from build123d import *

# Parameters (mm, degrees)
SKETCH1_W           = 4
SKETCH1_H           = 4
BOSS_EXTRUDE1_DEPTH = 12
CHAMFER3_SIZE       = 1
CHAMFER4_SIZE       = 1


with BuildPart() as part:
    # Sketch1 → Boss-Extrude1 (new body)
    with BuildSketch(Plane(origin=(0, 0, 0), x_dir=(1, 0, 0), z_dir=(0, 1, 0))):
        Rectangle(SKETCH1_W, SKETCH1_H)
    extrude(amount=BOSS_EXTRUDE1_DEPTH)

    # Chamfer3
    chamfer3_edges = [part.edges().sort_by_distance(p)[0] for p in [
        (-2, 12, 0),
        (0, 12, 2),
        (2, 12, 0),
        (0, 12, -2),
    ]]
    chamfer(chamfer3_edges, length=CHAMFER3_SIZE)

    # Chamfer4
    chamfer4_edges = [part.edges().sort_by_distance(p)[0] for p in [
        (0, 0, 2),
        (-2, 0, 0),
        (0, 0, -2),
        (2, 0, 0),
    ]]
    chamfer(chamfer4_edges, length=CHAMFER4_SIZE)


solid = part.part
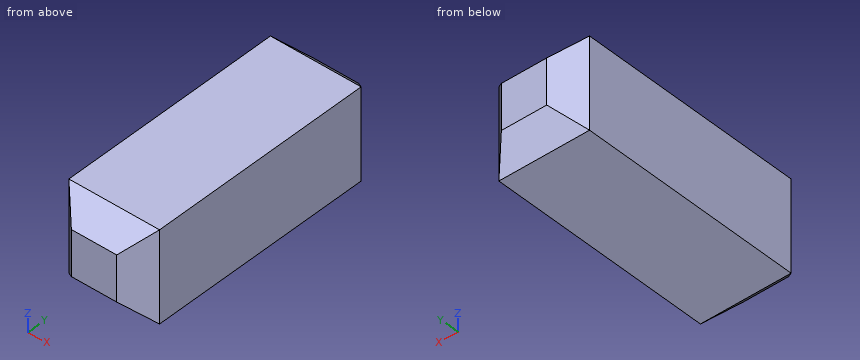
Read the model definition and answer for the solid it produces. Units are mm, in the model's axes. Give positions to 0.01 mm unless a question says otherwise; leave off trailing zeros. Loops run counter-clockwise (first coordinate to the right, second up) from the corner with the lowest first, then second, coordinate; pieces in that order, holes last. Notation, with made-up numbers: (70, 21.25) -> (84, 21.25) arc R36 ccw to (84, 56.25) -> close; hole circle Ø2 at (0.25, -11). An arc over 180 degrees is marked (long way). Answer as CSV lines item,"result".
Item 1: Consider line 1 (Y direction, x = -1.1, z = 0.1); line 2 (Y direction, x = 1, z = 1.7); line 3 (Z direction, x = 1.3, y = 11.5). Determine where each line is inside the solid, lowest interval first. Write a range as [from, to].
Returned:
line 1,"y = [0.1, 11.9]"
line 2,"y = [0.7, 11.3]"
line 3,"z = [-1.5, 1.5]"
Item 2: Find section A-A on x = 1.25. Give the vertices of the cut face in (y, z).
Returned:
outline,"(0.25, -1.25) -> (1, -2) -> (11, -2) -> (11.75, -1.25) -> (11.75, 1.25) -> (11, 2) -> (1, 2) -> (0.25, 1.25) -> close"
Item 3: Find section B-B on z = -1.2. Give the vertices of the cut face in (x, y).
Returned:
outline,"(-2, 1) -> (-1.2, 0.2) -> (1.2, 0.2) -> (2, 1) -> (2, 11) -> (1.2, 11.8) -> (-1.2, 11.8) -> (-2, 11) -> close"
